Geometry: final body of the model. Coordinates: model frame, mm. A direction names the side the tool comes from. Round coordinates to 2 decimals unless told otherwise and drop trailing zeros. Loops run counter-clockwise (first coordinate to the right, second up) from the corner with the lowest first, then second, coordinate; pieces in that order, holes last. Notation, with made-up numbers: (-12, 46.25) - (45, 46.25) arc R12 ccw to (45, 53.25) - close; hole circle Ø2 at (-31, 21). An arc over 180 degrees is marked (long way). Answer as a JSON object with one key per item and string values. Group by question number.
Item 1: Line query: line 1 (Y direction, x = 15.75, z = -9); line 2 (Z direction, x = 8.75, y = -2); line 3 (X direction, y = -1.5, z = -8.75). Output: solid intervals per line, ascending.
Item 2: First-contact query: pin 1 (3 mm diameter, centred on y = 0.5, z = -10, fed in from -X); pin 2 (0.7 mm diameter, centred on x = 5.5, z = -9.5, fed in from -Y); pin 3 (1 mm diameter, centred on x = 6.5, z = -8.5, fed in from +Y). Flat tips, straight axial feed; report the tip coordinate or a pass-through.
Item 3: Section A-A (x = 0). Return the cut outline in (y, z), plus the area to 3 significant figures.
Item 4: Section C-C (z = -10.75). Return the cut outline in (x, y).
Item 5: Section B-B (y = 0). Return the cut outline in (x, z).
Item 6: Draft query along Z for faces 1 (the face through (-3.1, 0, -9)), 2 (the face through (-0.07, -1.5, -4.69)), 3 (the face through (7, 0, -7.6)), 4 (the face through (0, 0, 0)). Return one class per face: released by +Z, released by -Z, zero draft, split by the parting line, or undercut.
Item 7: Section D-D (x = 12). Return the cut outline in (y, z).
Item 8: Reachability of faces 5 (the face through (-0.07, -1.5, -12.54)), 6 (the face through (0, 0, -15)) from +Z, -Z, +X, -X, +Y, -Y: full face, straight path, thin tool, end or side. Return the list, or none.
```python
from build123d import *

# Parameters (mm, degrees)
BOX_W     = 20
BOX_H     = 5.5
BOX_DEPTH = 2.4


with BuildPart() as nutslot:
    # Box → Box (new body)
    with BuildSketch(Plane(origin=(-3.1, -2.75, -10), x_dir=(1, 0, 0), z_dir=(0, 0, 1))):
        with Locations((10, 2.75)):
            Rectangle(BOX_W, BOX_H)
    extrude(amount=BOX_DEPTH)


with BuildPart() as countersunkcut:
    # Sketch007 → Revolution001 (revolve)
    with BuildSketch(Plane.YZ):
        Polygon((3.2, 0), (1.5, -1.7), (1.5, -15), (0, -15), (0, 0), align=None)
    revolve(axis=Axis((0, 0, 0), (0, 0, 1)))

    # Fusion: union NutSlot
    add(nutslot.part)


solid = countersunkcut.part
```
Values:
{
 "1": {"line 1": "y = -2.75 to 2.75", "line 2": "z = -10 to -7.6", "line 3": "x = -3.1 to 16.9"},
 "2": {"pin 1": "stops at x = -3.1", "pin 2": "stops at y = -2.75", "pin 3": "stops at y = 2.75"},
 "3": {"outline": "(-3.2, 0) - (-1.5, -1.7) - (-1.5, -7.6) - (-2.75, -7.6) - (-2.75, -10) - (-1.5, -10) - (-1.5, -15) - (1.5, -15) - (1.5, -10) - (2.75, -10) - (2.75, -7.6) - (1.5, -7.6) - (1.5, -1.7) - (3.2, 0) - close", "area": "53.9 mm^2"},
 "4": {"outline": "circle Ø3 at (0, 0)"},
 "5": {"outline": "(-3.2, 0) - (-1.5, -1.7) - (-1.5, -7.6) - (-3.1, -7.6) - (-3.1, -10) - (-1.5, -10) - (-1.5, -15) - (1.5, -15) - (1.5, -10) - (16.9, -10) - (16.9, -7.6) - (1.5, -7.6) - (1.5, -1.7) - (3.2, 0) - close"},
 "6": {"face 1": "zero draft", "face 2": "undercut", "face 3": "undercut", "face 4": "released by +Z"},
 "7": {"outline": "(-2.75, -10) - (2.75, -10) - (2.75, -7.6) - (-2.75, -7.6) - close"},
 "8": {"face 5": "-Z", "face 6": "-Z, +X, -X, +Y, -Y"}
}
